```python
from build123d import *

# Parameters (mm, degrees)
F0_R     = 5
F0_W     = 5
F0_H     = 20
F1_DEPTH = 5


with BuildPart() as f1:
    # F0 (on Front) → F1 (new body)
    with BuildSketch(Plane.XZ):
        with BuildLine():
            Line((41.89272, -49.099528), (110, -49.099528))
            Line((110, -49.099528), (115, -49.099528))
            Line((115, -49.099528), (115, -29.099528))
            Line((115, -29.099528), (110, -29.099528))
            Line((110, -29.099528), (110, -9.099528))
            Line((110, -9.099528), (115, -9.099528))
            Line((115, -9.099528), (115, 10.900472))
            Line((115, 10.900472), (110, 10.900472))
            Line((110, 10.900472), (110, 30.900472))
            Line((110, 30.900472), (115, 30.900472))
            Line((115, 30.900472), (115, 45.900472))
            Line((115, 45.900472), (69, 45.900472))
            Line((69, 45.900472), (69, 50.900472))
            Line((69, 50.900472), (23, 50.900472))
            Line((23, 50.900472), (23, 45.900472))
            Line((23, 45.900472), (-23, 45.900472))
            Line((-23, 45.900472), (-23, 50.900472))
            Line((-23, 50.900472), (-69, 50.900472))
            Line((-69, 50.900472), (-69, 45.900472))
            Line((-69, 45.900472), (-115, 45.900472))
            Line((-115, 45.900472), (-120, 45.900472))
            Line((-120, 45.900472), (-120, -49.099528))
            Line((-120, -49.099528), (-115, -49.099528))
            Line((-115, -49.099528), (-110, -49.099528))
            Line((-110, -49.099528), (-41.89272, -49.099528))
            ThreePointArc((-41.89272, -49.099528), (0, -22.099528), (41.89272, -49.099528))
        make_face()
        Polygon((-110, -29.099528), (-115, -29.099528), (-115, -9.099528), (-110, -9.099528), (-110, -19.099528), align=None, mode=Mode.SUBTRACT)
        with Locations((-95, 10.900472)):
            Circle(F0_R, mode=Mode.SUBTRACT)
        with Locations((-112.5, 20.900472)):
            Rectangle(F0_W, F0_H, mode=Mode.SUBTRACT)
    extrude(amount=F1_DEPTH)


solid = f1.part
```
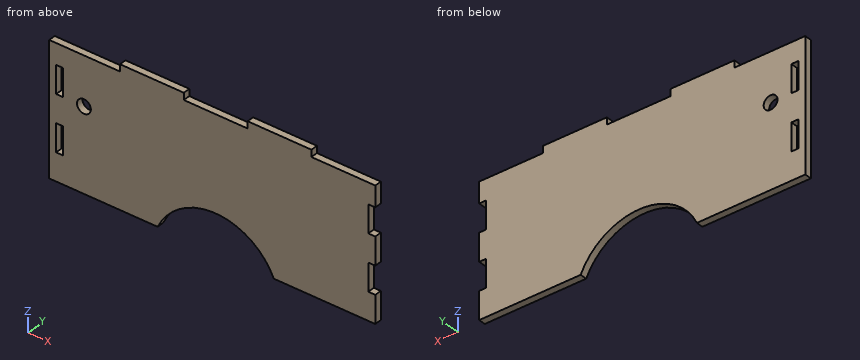
Check sheet for the modelled part. Datum: model origin and axes. Units: mm. Give positions to 0.01 mm unless a question says otherwise; leave off trailing zeros. Write each loop counter-clockwise with the first axis right and the second up, starting at its lowest first coordinate (ties: lowest second). Pieces come first, ordered by that corner, then holes.
Item 1: Cross-section at B-B (y = -2.85). Count the separate pieces of the cut face and the enclosed holes in it, and give its area (3 significant figures).
Item 2: Scan lines: L1, parallel to X at y = -1.7, z = 29; L2, parallel to Z at x = -95, y = -2.8; L3, parallel to X at y = -2.9, z = -27.5. Record each from-to range of solid material in increasing order.
Item 3: Cross-section at A-A (x = -95). Enter the section's corners in (y, z).
Item 4: Gauge pin test, flat ends, axial feed: pin 1 (2 mm diameter, centred on x = 80.5, y = -3, fed in from +Z); pin 2 (2.5 mm diameter, centred on y = -3, z = 49.5, fed in from +X); pin 3 (2.5 mm diameter, centred on y = -1.5, z = 49, fed in from -X). Record the tip position at first contact, or that the pin passes through.
Item 5: Cross-section at C-C (z = -24.5). Enter the section's corners in (x, y).
Report:
1. separate pieces: 1
1. enclosed holes: 3
1. area: 20,700 mm2
2. L1: x = -120 to -115, -110 to 110
2. L2: z = -49.1 to 5.9, 15.9 to 45.9
2. L3: x = -120 to -115, -110 to -21.63, 21.63 to 110
3. outline: (-5, -49.1) - (0, -49.1) - (0, 5.9) - (-5, 5.9) - close; (-5, 15.9) - (0, 15.9) - (0, 45.9) - (-5, 45.9) - close
4. pin 1: stops at z = 45.9
4. pin 2: stops at x = 69
4. pin 3: stops at x = -69
5. outline: (-120, -5) - (-115, -5) - (-115, 0) - (-120, 0) - close; (-110, -5) - (-14.67, -5) - (-14.67, 0) - (-110, 0) - close; (14.67, -5) - (110, -5) - (110, 0) - (14.67, 0) - close
